The listing builds one solid part. Answer for the finished solid, in the listing's coordinates (mm). A direction names the side the tool comes from. Give positions to 0.01 mm unless a question says otherwise; leave off trailing zeros. Write each loop counter-clockwise with the first axis right and the second up, starting at its lowest first coordinate (ties: lowest second). Pieces come first, ordered by that corner, then holes. Notation, with made-up numbers: (27.25, 62.25) - (69.25, 62.25) arc R21 ccw to (69.25, 80.25) - close; hole circle Ø6 at (38, 41.5). An arc over 180 degrees is marked (long way). Write each question's results on one line, items separated by ' | '. Start each with the question number.
Q1. For a pull along X with two mould halves and no side action, classify faces 5 (the face through (80, 0, -12)), 6 (the face through (1, 3, -15)), 7 (the face through (-6, -5, 44)) as pulls with the +X half, pulls with the -X half, needs draft (parallel to the pull), parting line crosses it, or undercut.
Q2. Flat-ended cylindrical pins translate along their axes: pin 1 Ø11 at (x, z) = (1.5, 64) entering from +Y; pin 2 Ø2 at (y, z) = (0, 67) entering from -X; pin 3 Ø24.5 at (y, z) = (19, 22) entering from +X. Find the tip coordinate at first contact, or state that the pin passes through.
Q3. For faces 1 (the face through (9, -6, 43)), 2 (the face through (0, -6, 46)), 3 (the face through (0, 8, 70)), 4 (the face through (43, 0, -7)), determine the directions among +Z, -Z, +X, -X, +Y, -Y from which every point of the face is accessible in a straight line to the end or side of a thin tool.
Q4. Section A-A (z = 74) is taken. Determine the outline of the cut face in (x, y), plus the area to 3 significant figures.
Q5. Section B-B (x = -30) is taken. Determine the outline of the cut face in (y, z), plus the area to 3 significant figures.
Q6. Find the intervals of material crossed by probe 1 along Z at (x, y) = (47, 6); probe 2 along X at (y, z) = (3.5, -1.5); probe 3 along Z at (x, y) = (39, 3.5), in increasing order.
```python
from build123d import *

# Parameters (mm, degrees)
F0_W          = 20
F0_H          = 16
F1_DEPTH      = 100
F1_DEPTH_BACK = 15
F2_T          = -2
F3_R          = 6.65
F4_DEPTH      = 25
F9_DEPTH      = 20
F10_R         = 5


with BuildPart() as f1:
    # F0 (on Top) → F1 (new body, two sides)
    with BuildSketch(Plane.XY) as f1_sk:
        Rectangle(F0_W, F0_H)
    extrude(amount=F1_DEPTH)
    extrude(f1_sk.sketch, amount=-F1_DEPTH_BACK)

    # F2
    f2_openings = [f1.faces().sort_by_distance(p)[0] for p in [
        (0, 0, 100),
    ]]
    offset(amount=F2_T, openings=f2_openings)

    # F3 (on Top) → F4 (cut)
    with BuildSketch(Plane.XY):
        with Locations((-23, 31)):
            Circle(F3_R)
    extrude(amount=F4_DEPTH, mode=Mode.SUBTRACT)

    # F7: sweep along a path in F6
    with BuildLine(Plane(origin=(0, 0, -15), x_dir=(1, 0, 0), z_dir=(0, 0, -1))) as f7_path:
        Line((-80, 0), (80, 0))
    # F5 (on face) → F7 (sweep)
    with BuildSketch(Plane.YZ.offset(10)):
        with BuildLine():
            Line((-8, -15), (8, -15))
            ThreePointArc((8, -15), (0, -7), (-8, -15))
        make_face()
    sweep(path=f7_path.line)

    # F8 (on face) → F9 (join)
    with BuildSketch(Plane.YZ.offset(10)):
        with BuildLine():
            Line((8, 39.9389689904), (8, -15))
            Line((8, -15), (34.332793206, -15))
            add(Edge.make_bspline(
                [(8, 39.9389689904), (8.920262118, 31.8490776814), (10.8133224807, 17.1951366341), (17.1653233274, 4.3539788499), (28.0984148898, -7.9715894697), (34.332793206, -15)],
                knots=[0.0556572186, 0.0556572186, 0.0556572186, 0.0556572186, 0.3658143049, 0.6383682032, 1, 1, 1, 1], degree=3))
        make_face()
    extrude(amount=-F9_DEPTH)

    # F10
    f10_edges = [f1.edges().sort_by_distance(p)[0] for p in [
        (-8, -6, 45.145751),
        (8, -6, 45.145751),
        (10, -8, 42.5),
        (-10, -8, 42.5),
        (8, 6, 45.145751),
        (-8, 6, 45.145751),
        (10, 8, 69.969484),
        (-10, 8, 69.969484),
        (10, 14.887336, 9.5352),
        (-10, 14.887336, 9.5352),
    ]]
    fillet(f10_edges, radius=F10_R)


solid = f1.part
```
Answers below:
1) face 5: pulls with the +X half | face 6: needs draft | face 7: undercut
2) pin 1: stops at y = 8 | pin 2: stops at x = -10 | pin 3: stops at x = 9.91
3) face 1: +Z, +X, -Y | face 2: +Z | face 3: +Z, +X, -X, +Y | face 4: +Z, +X
4) outline: (-10, -3) arc R5 ccw to (-5, -8) - (5, -8) arc R5 ccw to (10, -3) - (10, 3) arc R5 ccw to (5, 8) - (-5, 8) arc R5 ccw to (-10, 3) - close; hole (-8, -1) arc R5 ccw to (-3, -6) - (3, -6) arc R5 ccw to (8, -1) - (8, 1) arc R5 ccw to (3, 6) - (-3, 6) arc R5 ccw to (-8, 1) - close | area: 128 mm2
5) outline: (-8, -15) - (8, -15) arc R8 ccw to start | area: 101 mm2
6) probe 1: z = -15 to -9.71 | probe 2: x = -10 to -7.33, 7.33 to 10 | probe 3: z = -15 to -7.81
